```python
from build123d import *

# Parameters (mm, degrees)
BOSS_EXTRU_1_DEPTH      = 6
ESQUISSE2_R             = 1.5
ENL_V_MAT_EXTRU_1_DEPTH = 12
ESQUISSE3_R             = 1.5
ENL_V_MAT_EXTRU_2_DEPTH = 12
CONG_1_R                = 2
ENL_V_MAT_EXTRU_3_DEPTH = 3
ENL_V_START             = -3
ENL_V_MAT_EXTRU_4_DEPTH = 10


with BuildPart() as part:
    # Esquisse1 → Boss.-Extru.1 (new, symmetric)
    with BuildSketch(Plane(origin=(0, 0, 0), x_dir=(1, 0, 0), z_dir=(0, 1, 0))):
        with BuildLine():
            Line((-12, 0), (0, 0))
            Line((0, 0), (0, -66))
            ThreePointArc((0, -66), (-2.636038969, -72.363961031), (-9, -75))
            Line((-9, -75), (-74, -75))
            Line((-74, -75), (-74, -73.5))
            Line((-74, -73.5), (-87, -73.5))
            Line((-87, -73.5), (-87, -67.5))
            Line((-87, -67.5), (-74, -67.5))
            Line((-74, -67.5), (-66.205771366, -72))
            Line((-66.205771366, -72), (-9, -72))
            ThreePointArc((-9, -72), (-4.757359313, -70.242640687), (-3, -66))
            Line((-3, -66), (-3, -9.196152423))
            Line((-3, -9.196152423), (-12, -4))
            Line((-12, -4), (-12, 0))
        make_face()
    extrude(amount=BOSS_EXTRU_1_DEPTH, both=True)

    # Esquisse2 → Enlèv. mat.-Extru.1 (cut)
    with BuildSketch(Plane(origin=(0, 0, 0), x_dir=(-1, 0, 0), z_dir=(0, 0, -1))):
        with Locations((6, 0)):
            Circle(ESQUISSE2_R)
    extrude(amount=-ENL_V_MAT_EXTRU_1_DEPTH, mode=Mode.SUBTRACT)

    # Esquisse3 → Enlèv. mat.-Extru.2 (cut)
    with BuildSketch(Plane(origin=(0, 0, 67.5), x_dir=(-1, 0, 0), z_dir=(0, 0, -1))):
        with Locations((81, 0)):
            Circle(ESQUISSE3_R)
    extrude(amount=-ENL_V_MAT_EXTRU_2_DEPTH, mode=Mode.SUBTRACT)

    # Congé1
    cong_1_edges = [part.edges().sort_by_distance(p)[0] for p in [
        (-87, 0, 73.5),
        (-87, 0, 67.5),
        (-74, 0, 67.5),
        (-66.205771366, 0, 72),
        (-3, 0, 9.196152423),
        (-12, 0, 4),
    ]]
    fillet(cong_1_edges, radius=CONG_1_R)

    # Esquisse4 → Enlèv. mat.-Extru.3 (cut)
    with BuildSketch(Plane(origin=(0, 0, 67.5), x_dir=(-1, 0, 0), z_dir=(0, 0, -1))):
        Polygon((83.8, 1.616580754), (81, 3.233161507), (78.2, 1.616580754), (78.2, -1.616580754), (81, -3.233161507), (83.8, -1.616580754), align=None)
    extrude(amount=-ENL_V_MAT_EXTRU_3_DEPTH, mode=Mode.SUBTRACT)

    # Esquisse5 → Enlèv. mat.-Extru.4 (cut)
    with BuildSketch(Plane(origin=(0, 0, 0), x_dir=(-1, 0, 0), z_dir=(0, 0, -1)).offset(ENL_V_START)):
        Polygon((8.8, 1.616580754), (6, 3.233161507), (3.2, 1.616580754), (3.2, -1.616580754), (6, -3.233161507), (8.8, -1.616580754), align=None)
    extrude(amount=-ENL_V_MAT_EXTRU_4_DEPTH, mode=Mode.SUBTRACT)


solid = part.part
```
Design review of the part built by this model. Coordinates are the model's own, in mm. A direction names the side the tool comes from. Give positions to 0.01 mm unless a question says otherwise; leave off trailing zeros. Write each loop counter-clockwise with the first axis right and the second up, starting at its lowest first coordinate (ties: lowest second). Pieces come first, ordered by that corner, then holes. Notation, with made-up numbers: (28, 26) -> (38, 26) arc R23 ccw to (38, 61) -> close; hole circle Ø7 at (-20.5, 50.5). An arc over 180 degrees is marked (long way). Answer in a Markdown table with one row per item.
(1) Mouldability with a two-part tool opening along X and no side actions: class faces 1 (the flat face through (-79, 0, 73.5)), 2 (the cylindrical face through (-86.4, -0.08, 72.93)), 3 (the flat face through (-8.8, 0, 4)) as +X half, -X half, draft (parallel to the pull), parting line (faces both ways), or undercut.
Results:
| item | result |
|---|---|
| face 1 | draft |
| face 2 | -X half |
| face 3 | undercut |
(2) Clearance check with flat-ended pins moving along their axes: pin 1 (3.5 mm diameter, centred on y = 0, z = 69, fed in from +X); pin 2 (6 mm diameter, centred on x = -80, y = -0.5, fed in from -Z); pin 3 (3 mm diameter, centred on y = 1, z = 2, fed in from -X). State where each tip first meets the part, or that it passes through.
Results:
| item | result |
|---|---|
| pin 1 | x = -0.09 |
| pin 2 | z = 67.5 |
| pin 3 | x = -12 |
(3) Consider section B-B (x = -46). State the section outline as (y, z) points, then the cut area to 3 significant figures.
Results:
| item | result |
|---|---|
| outline | (-6, 72) -> (6, 72) -> (6, 75) -> (-6, 75) -> close |
| area | 36.0 mm2 |
(4) Consider section C-C (z = 26). State the section outline as (x, y) points.
Results:
| item | result |
|---|---|
| outline | (-3, -6) -> (0, -6) -> (0, 6) -> (-3, 6) -> close |
(5) To check wall thickness, follow probe 1 along X at (y, z) = (3, 68); probe 2 along Y at (x, z) = (-81, 71); probe 3 along Z at (x, y) = (-54, -2.25). State the ranges of each line that lie inside material, in increasing order.
Results:
| item | result |
|---|---|
| probe 1 | -86.32 to -81.4, -80.6 to -73.13, -3.34 to -0.23 |
| probe 2 | -6 to -1.5, 1.5 to 6 |
| probe 3 | 72 to 75 |
(6) Consider section A-A (y = 0). Count the separate pieces of the cut face and the enclosed holes in it, then the cut area to 3 significant figures.
Results:
| item | result |
|---|---|
| separate pieces | 3 |
| enclosed holes | 0 |
| area | 522 mm2 |
(7) For faces 4 (the flat face through (-3, 0, 39)), 5 (the flat face through (-78.2, 0, 69)), 6 (the cylindrical face through (-4.804, 0.084, 70.289)), list the 3-axis set-ups (+Z, -Z, +X, -X, +Y, -Y) from which the entire face can be reached by the end or side of a thin tool; tool diameter is ignored.
Results:
| item | result |
|---|---|
| face 4 | -X, +Y, -Y |
| face 5 | -Z |
| face 6 | +Y, -Y |
